Work out the finished part from the listing and answer in its coordinate system (mm). Face numbers are marked on the shaded views. A direction names the side the tool comes from. Coordinates: 2 decimals unless noted, no trailing zeros. Write each loop counter-clockwise with the first axis right and the second up, starting at its lowest first coordinate (ties: lowest second). Pieces come first, ordered by that corner, then holes. Notation, with made-up numbers: M 37,0.25 L 49,0.25 A8 ccw 49,7.25 Z; hole C 5,5.25 d1. An arc over 180 degrees is marked long. Answer as CSV lines item,"result". Start each with the question number.
(1) Find the intervals of material crossed by L1, parallel to Y at x = 0, z = -0.35; L2, parallel to Y at x = 0, z = -2.4; L3, parallel to Y at x = -0.5, z = -0.95, in increasing order. Write a range as [from, to].
(2) Flat-ended cylindrical pins translate along their axes: P1, Ø2, axis at y = -2, z = 0.5, coming from the -X side; P2, Ø1.5, axis at x = -5, z = -1, coming from the -Y side; P3, Ø1.5, axis at y = 3.5, z = 1, coming from the -X side; P4, Ø4, axis at x = 0, y = 0, coming from the -Z side. Find the tip coordinate at first contact, or state that the pin passes through.
(3) The mould has two halves that part along Y. Classify the marked faces 3, 4 and 5: released by +Y, released by -Y, zero draft, split by the parting line, or undercut.
(4) A cutting plane is placed at A-A on z = 2.05. Give the vertices of the cut face in (x, y), then the cut area to 3 significant figures.
(5) For the marked faces 1 and 2, determine the directions among +Z, -Z, +X, -X, +Y, -Y from which every point of the face is accessible in a straight line to the end or side of a thin tool.
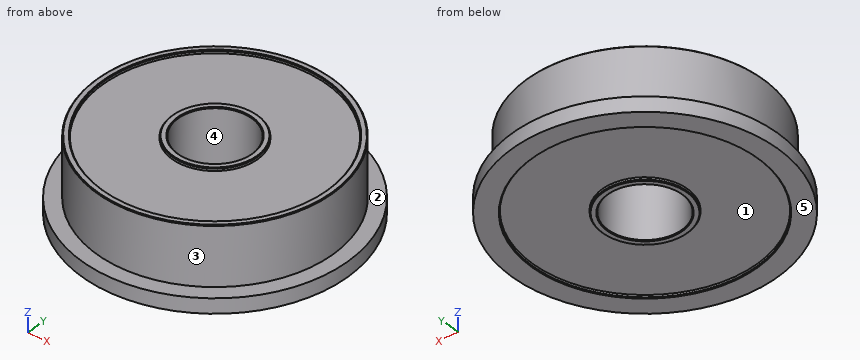
from build123d import *

# Parameters (mm, degrees)
SKETCH_1_R          = 8
SKETCH_1_R_2        = 2.5
EXTRUDE_1_DEPTH     = 2.5
SKETCH_3_R          = 9
SKETCH_3_R_2        = 2.5
EXTRUDE_2_DEPTH     = 1
SKETCH_4_R          = 7.6
SKETCH_4_R_2        = 2.9
CUT_EXTRUDE_1_DEPTH = 0.2
CHAMFER_1_SIZE      = 0.05


with BuildPart() as part:
    # 草图1 → 凸台-拉伸1 (new, symmetric)
    with BuildSketch(Plane.XY):
        Circle(SKETCH_1_R)
        Circle(SKETCH_1_R_2, mode=Mode.SUBTRACT)
    extrude(amount=EXTRUDE_1_DEPTH, both=True)

    # 草图3 → 凸台-拉伸2 (add)
    with BuildSketch(Plane(origin=(0, 0, -2.5), x_dir=(-1, 0, 0), z_dir=(0, 0, -1))):
        Circle(SKETCH_3_R)
        with Locations(Location((0, 0, 0), (0, 0, 180))):
            Circle(SKETCH_3_R_2, mode=Mode.SUBTRACT)
    extrude(amount=-EXTRUDE_2_DEPTH)

    # 草图4 → 切除-拉伸1 (cut)
    with BuildSketch(Plane.XY.offset(2.5)):
        Circle(SKETCH_4_R)
        Circle(SKETCH_4_R_2, mode=Mode.SUBTRACT)
    cut_extrude_1 = extrude(amount=-CUT_EXTRUDE_1_DEPTH, mode=Mode.SUBTRACT)

    # 镜向1: 切除-拉伸1 across plane
    add(cut_extrude_1.mirror(Plane.XY), mode=Mode.SUBTRACT)

    # 倒角1
    chamfer_1_edges = [part.edges().sort_by_distance(p)[0] for p in [
        (-7.6, 0, 2.5),
        (-2.9, 0, 2.5),
        (-2.9, 0, -2.5),
        (-7.6, 0, -2.5),
        (-8, 0, 2.5),
        (-2.5, 0, -2.5),
        (-2.5, 0, 2.5),
    ]]
    chamfer(chamfer_1_edges, length=CHAMFER_1_SIZE)


solid = part.part
Here are the results:
1,L1,"y = [-8, -2.5], [2.5, 8]"
1,L2,"y = [-9, -7.6], [-2.9, -2.5], [2.5, 2.9], [7.6, 9]"
1,L3,"y = [-7.98, -2.45], [2.45, 7.98]"
2,P1,"stops at x = -7.94"
2,P2,"stops at y = -7.83"
2,P3,"stops at x = -7.51"
2,P4,"passes through"
3,face 3,"split by the parting line"
3,face 4,"undercut"
3,face 5,"zero draft"
4,outline,"C 0,0 d16; hole C 0,0 d5"
4,area,"181 mm^2"
5,face 1,"-Z"
5,face 2,"+Z"
